The listing builds one solid part. Answer for the finished solid, in the listing's coordinates (mm). A direction names the side the tool comes from. Give positions to 0.01 mm unless a question says otherwise; leave off trailing zeros. Order: outer loops, then holes, each group sorted by start corner. A loop starts at its lowest first (then second) coordinate and runs counter-clockwise, first axis right, second up. Notation, with made-up numbers: M -32.5,85 L -27.5,85 A19 cw -27.5,105 Z; hole C 0.25,-8.75 d9. An arc over 180 degrees is marked long. Answer as a JSON object with one key per item and string values. Group by question number.
```python
from build123d import *

# Parameters (mm, degrees)
SKETCH2_R               = 20
SKETCH2_R_2             = 10
BOSS_EXTRUDE1_DEPTH     = 80
SKETCH3_R               = 20
BOSS_EXTRUDE2_DEPTH     = 5
SKETCH4_W               = 30
SKETCH4_H               = 30
CUT_EXTRUDE1_DEPTH      = 50
SKETCH4_4_W             = 40
SKETCH4_4_H             = 40
SKETCH4_4_W_2           = 30
SKETCH4_4_H_2           = 30
BOSS_EXTRUDE3_DEPTH     = 127
SKETCH4_5_W             = 30
SKETCH4_5_H             = 30
CUT_EXTRUDE2_DEPTH      = 10
SKETCH5_R               = 10
CUT_EXTRUDE3_DEPTH      = 50
BOSS_EXTRUDE4_DEPTH     = 245
SKETCH7_W               = 25
SKETCH7_H               = 5
SKETCH7_W_2             = 55.000380238
BOSS_EXTRUDE5_DEPTH     = 35
SKETCH11_W              = 65
SKETCH11_H              = 5
BOSS_EXTRUDE9_DEPTH     = 245
SKETCH9_W               = 40
SKETCH9_H               = 40
CUT_EXTRUDE4_DEPTH      = 10
SKETCH9_4_W             = 50
SKETCH9_4_H             = 50
SKETCH9_4_W_2           = 40
SKETCH9_4_H_2           = 40
BOSS_EXTRUDE10_DEPTH    = 116
SKETCH13_W              = 50
SKETCH13_H              = 50
BOSS_EXTRUDE11_DEPTH    = 5
SKETCH14_W              = 40
SKETCH14_H              = 40
CUT_EXTRUDE5_DEPTH      = 5
CUT_EXTRUDE6_DEPTH      = 393
SKETCH16_W              = 40
SKETCH16_H              = 35
CUT_EXTRUDE7_DEPTH      = 1
CUT_EXTRUDE7_DEPTH_BACK = 66


with BuildPart() as part:
    # Sketch2 → Boss-Extrude1 (new body)
    with BuildSketch(Plane(origin=(0, 0, 0), x_dir=(1, 0, 0), z_dir=(0, 1, 0))):
        Circle(SKETCH2_R)
        Circle(SKETCH2_R_2, mode=Mode.SUBTRACT)
    extrude(amount=BOSS_EXTRUDE1_DEPTH)

    # Sketch3 → Boss-Extrude2 (add)
    with BuildSketch(Plane(origin=(0, 80, 0), x_dir=(1, 0, 0), z_dir=(0, 1, 0))):
        Circle(SKETCH3_R)
    extrude(amount=BOSS_EXTRUDE2_DEPTH)

    # Sketch4 → Cut-Extrude1 (cut)
    with BuildSketch(Plane.XY):
        with Locations((0, 65)):
            Rectangle(SKETCH4_W, SKETCH4_H)
    extrude(amount=-CUT_EXTRUDE1_DEPTH, mode=Mode.SUBTRACT)

    # Sketch4<4> → Boss-Extrude3 (add)
    with BuildSketch(Plane.XY):
        with Locations((0, 65)):
            Rectangle(SKETCH4_4_W, SKETCH4_4_H)
        with Locations((0, 65)):
            Rectangle(SKETCH4_4_W_2, SKETCH4_4_H_2, mode=Mode.SUBTRACT)
    extrude(amount=-BOSS_EXTRUDE3_DEPTH)

    # Sketch4<5> → Cut-Extrude2 (cut)
    with BuildSketch(Plane.XY):
        with Locations((0, 65)):
            Rectangle(SKETCH4_5_W, SKETCH4_5_H)
    extrude(amount=CUT_EXTRUDE2_DEPTH, mode=Mode.SUBTRACT)

    # Sketch5 → Cut-Extrude3 (cut)
    with BuildSketch(Plane.XZ):
        Circle(SKETCH5_R)
    extrude(amount=-CUT_EXTRUDE3_DEPTH, mode=Mode.SUBTRACT)

    # Sketch6 → Boss-Extrude4 (add)
    with BuildSketch(Plane(origin=(0, 0, -127), x_dir=(-1, 0, 0), z_dir=(0, 0, -1))):
        Polygon((0, 80), (0, 85), (20, 85), (20, 45), (-45, 45), (-45, 85), (-40, 85), (-40, 49.795485049), (15, 50), (15, 80), align=None)
    extrude(amount=BOSS_EXTRUDE4_DEPTH)

    # Sketch7 → Boss-Extrude5 (add)
    with BuildSketch(Plane(origin=(0.185712712, 49.943532631, 0), x_dir=(0.999993087, -0.003718428, 0), z_dir=(0.003718428, 0.999993087, 0))):
        with Locations((27.314562541, 129.5)):
            Rectangle(SKETCH7_W, SKETCH7_H)
        with Locations((12.314372422, 369.5)):
            Rectangle(SKETCH7_W_2, SKETCH7_H)
    extrude(amount=BOSS_EXTRUDE5_DEPTH)

    # Sketch11 → Boss-Extrude9 (add)
    with BuildSketch(Plane(origin=(0, 0, -372), x_dir=(-1, 0, 0), z_dir=(0, 0, -1))):
        with Locations((-12.5, 82.5)):
            Rectangle(SKETCH11_W, SKETCH11_H)
    extrude(amount=-BOSS_EXTRUDE9_DEPTH)

    # Sketch9 → Cut-Extrude4 (cut)
    with BuildSketch(Plane(origin=(0, 85, 0), x_dir=(1, 0, 0), z_dir=(0, 1, 0))):
        with Locations((20, 152)):
            Rectangle(SKETCH9_W, SKETCH9_H)
        with Locations((20, 217)):
            Rectangle(SKETCH9_W, SKETCH9_H)
        with Locations((20, 282)):
            Rectangle(SKETCH9_W, SKETCH9_H)
        with Locations((20, 347)):
            Rectangle(SKETCH9_W, SKETCH9_H)
    extrude(amount=-CUT_EXTRUDE4_DEPTH, mode=Mode.SUBTRACT)

    # Sketch9<4> → Boss-Extrude10 (add)
    with BuildSketch(Plane(origin=(0, 85, 0), x_dir=(1, 0, 0), z_dir=(0, 1, 0))):
        with Locations((20, 152)):
            Rectangle(SKETCH9_4_W, SKETCH9_4_H)
        with Locations((20, 152)):
            Rectangle(SKETCH9_4_W_2, SKETCH9_4_H_2, mode=Mode.SUBTRACT)
        with Locations((20, 217)):
            Rectangle(SKETCH9_4_W, SKETCH9_4_H)
        with Locations((20, 217)):
            Rectangle(SKETCH9_4_W_2, SKETCH9_4_H_2, mode=Mode.SUBTRACT)
        with Locations((20, 282)):
            Rectangle(SKETCH9_4_W, SKETCH9_4_H)
        with Locations((20, 282)):
            Rectangle(SKETCH9_4_W_2, SKETCH9_4_H_2, mode=Mode.SUBTRACT)
        with Locations((20, 347)):
            Rectangle(SKETCH9_4_W, SKETCH9_4_H)
        with Locations((20, 347)):
            Rectangle(SKETCH9_4_W_2, SKETCH9_4_H_2, mode=Mode.SUBTRACT)
    extrude(amount=BOSS_EXTRUDE10_DEPTH)

    # Sketch13 → Boss-Extrude11 (add)
    with BuildSketch(Plane(origin=(0, 201, 0), x_dir=(1, 0, 0), z_dir=(0, 1, 0))):
        with Locations((20, 152)):
            Rectangle(SKETCH13_W, SKETCH13_H)
        with Locations((20, 217)):
            Rectangle(SKETCH13_W, SKETCH13_H)
        with Locations((20, 282)):
            Rectangle(SKETCH13_W, SKETCH13_H)
        with Locations((20, 347)):
            Rectangle(SKETCH13_W, SKETCH13_H)
    extrude(amount=BOSS_EXTRUDE11_DEPTH)

    # Sketch14 → Cut-Extrude5 (cut)
    with BuildSketch(Plane.ZY.offset(5)):
        with Locations((-347, 181)):
            Rectangle(SKETCH14_W, SKETCH14_H)
        with Locations((-282, 181)):
            Rectangle(SKETCH14_W, SKETCH14_H)
        with Locations((-217, 181)):
            Rectangle(SKETCH14_W, SKETCH14_H)
        with Locations((-152, 181)):
            Rectangle(SKETCH14_W, SKETCH14_H)
    extrude(amount=-CUT_EXTRUDE5_DEPTH, mode=Mode.SUBTRACT)

    # Sketch15 → Cut-Extrude6 (cut, through all)
    with BuildSketch(Plane(origin=(0, 0, -372), x_dir=(-1, 0, 0), z_dir=(0, 0, -1))):
        Polygon((-20, 206), (5, 161), (5, 206), align=None)
    extrude(amount=-CUT_EXTRUDE6_DEPTH, mode=Mode.SUBTRACT)

    # Sketch16 → Cut-Extrude7 (cut, two sides)
    with BuildSketch(Plane.ZY.offset(20)) as cut_extrude7_sk:
        with Locations((0, 17.5)):
            Rectangle(SKETCH16_W, SKETCH16_H)
    extrude(amount=CUT_EXTRUDE7_DEPTH, mode=Mode.SUBTRACT)
    extrude(cut_extrude7_sk.sketch, amount=-CUT_EXTRUDE7_DEPTH_BACK, mode=Mode.SUBTRACT)


solid = part.part
```
Item 1: Section C-C (z = -292) is taken. Determine the outline of the cut face in (x, y).
Item 2: Section D-D (z = -58) is taken. Determine the outline of the cut face in (x, y), and give its area (3 significant figures).
Item 3: Flat-ended cylindrical pins translate along their axes: P1, Ø2, axis at x = -11.5, z = -309.5, coming from the +Y side; P2, Ø5, axis at x = 32, y = 180.5, coming from the +Z side; P3, Ø7, axis at x = 25, z = -273, coming from the -Y side. Find the tip coordinate at first contact, or state that the pin passes through.
Item 4: Section A-A (y = 188) is taken. Count the separate pieces of the cut face and the enclosed holes in it, and give its area (3 significant figures).
Item 5: Determine the mould class of faces 1 (the flat face through (40, 124, -222)), 2 (the flat face through (-5, 122, -152)), 3 (the flat face through (19, 109, -372)), 4 (the flat face through (0, 121, -217)) for opening direction X: released by +X, released by -X, zero draft, split by the parting line, or undercut.
Item 6: Consider probe 1 along X at (y, z) = (127.5, -228); probe 2 along Z at (x, y) = (26.5, 54.5); probe 3 along Y at (x, z) = (29.5, -244.5). Determine where each line is inside the solid, lowest interval first. Write a range as from..to.
Item 7: A tool of negligible diameter and unlimited length cuts with its end or side. For faces 5 (the flat face through (20, 145, -257)), 6 (the cylindrical face through (-4.336, 54.094, 19.524)), 7 (the flat face through (22, 140, -262)), 8 (the flat face through (20, 65, -63)), from which of +Z, -Z, +X, -X, +Y, -Y can it reach the whole face along a straight path? Write none if from no direction.
Item 8: Section B-B (z = -181.5) is taken. Determine the outline of the cut face in (x, y).
Values found:
{
 "1": {"outline": "M -20,45 L 45,45 L 45,206 L 20,206 L 17.22,201 L 40,201 L 40,49.8 L -15,50 L -15,80 L 0,80 L 0,161 L -5,161 L -5,85 L -20,85 Z"},
 "2": {"outline": "M -20,45 L 20,45 L 20,85 L -20,85 Z; hole M -15,50 L 15,50 L 15,80 L -15,80 Z", "area": "700 mm^2"},
 "3": {"P1": "stops at y = 85", "P2": "stops at z = -127", "P3": "stops at y = 45"},
 "4": {"separate pieces": "4", "enclosed holes": "0", "area": "2,200 mm^2"},
 "5": {"face 1": "undercut", "face 2": "released by -X", "face 3": "zero draft", "face 4": "undercut"},
 "6": {"probe 1": "x = -5..0, 40..45", "probe 2": "z = -372..-367, -132..-127", "probe 3": "y = 45..49.83, 80..85"},
 "7": {"face 5": "+X, -X, +Y", "face 6": "-Y", "face 7": "none", "face 8": "+Z, +X, +Y, -Y"},
 "8": {"outline": "M -20,45 L 45,45 L 45,85 L -20,85 Z; hole M -15,50 L 40,49.8 L 40,80 L -15,80 Z"}
}
